Here's the drawing with two shaded views (mm, measured from the low corner). I have some questions. A direction names the side the tool comes from. Give positions to 0.01 mm unless a question says otherwise; leave off trailing zeros. Write each loop counter-clockwise with the first axis right and the second up, starting at its lowest first coordinate (ties: lowest second). Pieces come first, ordered by that corner, then holes.
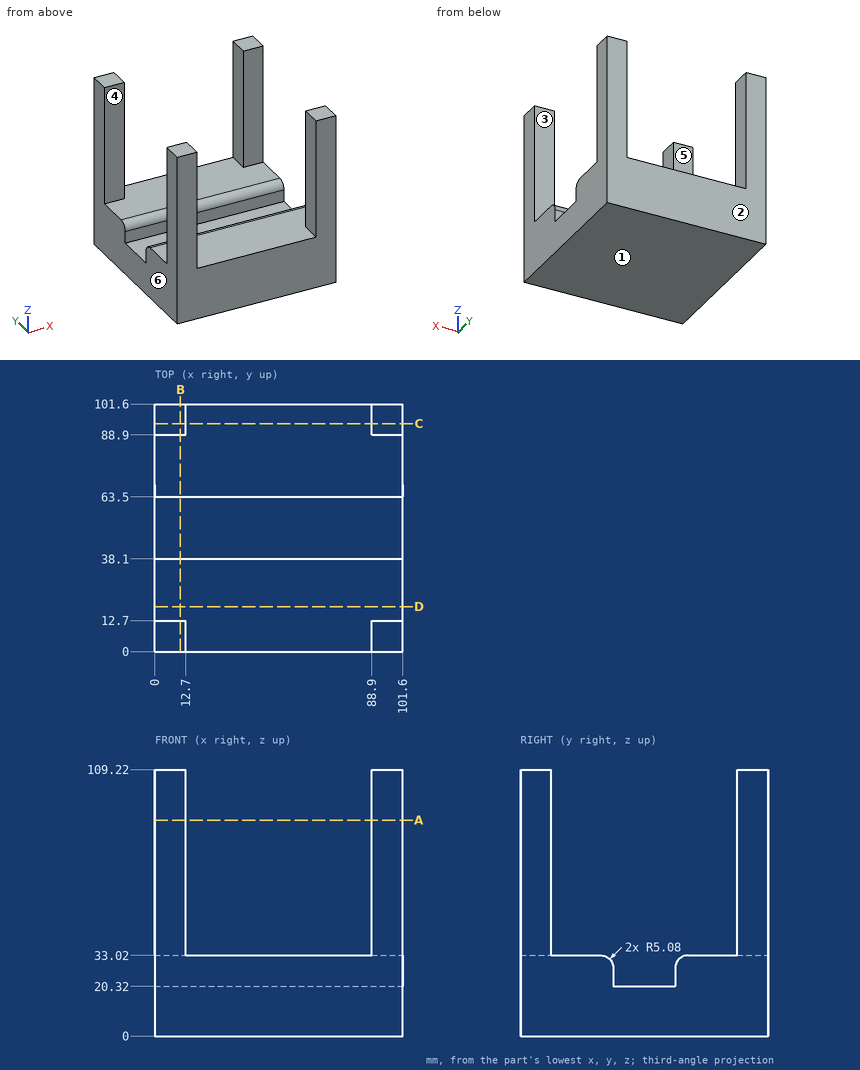
1) For the marked faces 5 and 6, which set-ups out of +Z, -Z, +X, -X, +Y, -Y let a thin tool reach every point of the face, with its end or its side?
Values follow:
face 5: +Z, +X, -X
face 6: +Z, -Z, -X, +Y, -Y
2) For pin 1 Ø10 at (x, y) = (91.5, 26.5) entering from +Z; pin 2 Ø20.5 at (x, y) = (57, 52) entering from +Z, each with a flat end and sliding along its axis, tell me the tip position at first contact or that it passes through.
Values follow:
pin 1: stops at z = 33.02
pin 2: stops at z = 20.32
3) Suppose I cut it at B-B on x = 10.5. Write out the boundary of the cut face in (y, z), plus the area to 3 significant figures.
Values follow:
outline: (0, 0) - (101.6, 0) - (101.6, 109.22) - (88.9, 109.22) - (88.9, 33.02) - (68.58, 33.02) arc R5.08 ccw to (63.5, 27.94) - (63.5, 20.32) - (38.1, 20.32) - (38.1, 27.94) arc R5.08 ccw to (33.02, 33.02) - (12.7, 33.02) - (12.7, 109.22) - (0, 109.22) - close
area: 4,960 mm2
4) Please list where these lines run through material, in increasing order: L1, parallel to X at y = 5.5, z = 95; L2, parallel to Z at x = 38, y = 45.5.
Values follow:
L1: x = 0 to 12.7, 88.9 to 101.6
L2: z = 0 to 20.32
5) Suppose I cut it at C-C on y = 93.5. Write out the boundary of the cut face in (x, z), plus the area to 3 significant figures.
Values follow:
outline: (0, 0) - (101.6, 0) - (101.6, 109.22) - (88.9, 109.22) - (88.9, 33.02) - (12.7, 33.02) - (12.7, 109.22) - (0, 109.22) - close
area: 5,290 mm2
6) Suppose I cut it at A-A on z = 88.5. Write out the boundary of the cut face in (x, y), plus the area to 3 significant figures.
Values follow:
outline: (0, 0) - (12.7, 0) - (12.7, 12.7) - (0, 12.7) - close; (0, 88.9) - (12.7, 88.9) - (12.7, 101.6) - (0, 101.6) - close; (88.9, 0) - (101.6, 0) - (101.6, 12.7) - (88.9, 12.7) - close; (88.9, 88.9) - (101.6, 88.9) - (101.6, 101.6) - (88.9, 101.6) - close
area: 645 mm2
7) Suppose I cut it at D-D on y = 18.5. Write out the boundary of the cut face in (x, z), plus the area to 3 significant figures.
Values follow:
outline: (0, 0) - (101.6, 0) - (101.6, 33.02) - (0, 33.02) - close
area: 3,350 mm2
8) If we mould it in two halves opening along Y, with no side actions, what happens to the marked faces 1, 2, 3 and 4? For each: +Y half, -Y half, draft (parallel to the pull), parting line (faces both ways), or undercut.
Values follow:
face 1: draft
face 2: +Y half
face 3: undercut
face 4: undercut
